```python
from build123d import *

# Parameters (mm, degrees)
BOSS_EXTRUDE1_DEPTH                             = 6.35
FILLET1_R                                       = 10
CSK_FOR_M4_FLAT_HEAD_MACHINE_SCREW1_D           = 4.5
CSK_FOR_M4_FLAT_HEAD_MACHINE_SCREW1_DEPTH       = 41.15
CSK_FOR_M4_FLAT_HEAD_MACHINE_SCREW1_CSINK_D     = 9.4
CSK_FOR_M4_FLAT_HEAD_MACHINE_SCREW1_CSINK_ANGLE = 90
CSK_FOR_M4_FLAT_HEAD_MACHINE_SCREW1_TIP         = 1.351936393
SKETCH5_R                                       = 23.5
CUT_EXTRUDE1_DEPTH                              = 91.971053662
FILLET2_R                                       = 5


with BuildPart() as part:
    # Sketch1 → Boss-Extrude1 (new body)
    with BuildSketch(Plane(origin=(0, 0, 0), x_dir=(1, 0, 0), z_dir=(0, 1, 0))):
        with BuildLine():
            ThreePointArc((-15.208520638, -24.071794541), (-40.946506862, -5.668779355), (-50.8, 24.398205459))
            Line((-50.8, 24.398205459), (-50.8, -73.601794541))
            Line((-50.8, -73.601794541), (-30.8, -73.601794541))
            Line((-30.8, -73.601794541), (-30.8, -24.071794541))
            Line((-30.8, -24.071794541), (-15.208520638, -24.071794541))
        make_face()
        with BuildLine():
            Line((0, 24.398205459), (-50.8, 24.398205459))
            ThreePointArc((-50.8, 24.398205459), (-40.946506862, -5.668779355), (-15.208520638, -24.071794541))
            Line((-15.208520638, -24.071794541), (0, -24.071794541))
            Line((0, -24.071794541), (0, 24.398205459))
        make_face()
        with BuildLine():
            Line((50.8, 24.398205459), (0, 24.398205459))
            Line((0, 24.398205459), (0, -24.071794541))
            Line((0, -24.071794541), (15.208520638, -24.071794541))
            ThreePointArc((15.208520638, -24.071794541), (40.946506862, -5.668779355), (50.8, 24.398205459))
        make_face()
        with BuildLine():
            ThreePointArc((50.8, 24.398205459), (0, 75.198205459), (-50.8, 24.398205459))
            Line((-50.8, 24.398205459), (0, 24.398205459))
            Line((0, 24.398205459), (50.8, 24.398205459))
        make_face()
        with BuildLine():
            Line((50.8, -73.601794541), (50.8, 24.398205459))
            ThreePointArc((50.8, 24.398205459), (40.946506862, -5.668779355), (15.208520638, -24.071794541))
            Line((15.208520638, -24.071794541), (30.8, -24.071794541))
            Line((30.8, -24.071794541), (30.8, -73.601794541))
            Line((30.8, -73.601794541), (50.8, -73.601794541))
        make_face()
    extrude(amount=BOSS_EXTRUDE1_DEPTH)

    # Fillet1
    fillet1_edges = [part.edges().sort_by_distance(p)[0] for p in [
        (-30.8, 3.175, 24.071794541),
        (30.8, 3.175, 24.071794541),
    ]]
    fillet(fillet1_edges, radius=FILLET1_R)

    # CSK for M4 Flat Head Machine Screw1
    with Locations(Plane.XZ):
        with Locations((44.261727213, -14.295755058), (-44.45, 65.601794541), (44.45, 65.601794541), (-44.45, 21.601794541), (44.45, 21.601794541), (19.698321756, 16.505781144), (-19.698321756, 16.505781144), (-44.261727213, -14.295755058), (-35.495149304, -52.704642464), (0, -69.798205459), (35.495149304, -52.704642464)):
            CounterSinkHole(CSK_FOR_M4_FLAT_HEAD_MACHINE_SCREW1_D / 2, CSK_FOR_M4_FLAT_HEAD_MACHINE_SCREW1_CSINK_D / 2, depth=CSK_FOR_M4_FLAT_HEAD_MACHINE_SCREW1_DEPTH, counter_sink_angle=CSK_FOR_M4_FLAT_HEAD_MACHINE_SCREW1_CSINK_ANGLE)
            with Locations((0, 0, -(CSK_FOR_M4_FLAT_HEAD_MACHINE_SCREW1_DEPTH + CSK_FOR_M4_FLAT_HEAD_MACHINE_SCREW1_TIP / 2))):  # 118° drill point
                Cone(0, CSK_FOR_M4_FLAT_HEAD_MACHINE_SCREW1_D / 2, CSK_FOR_M4_FLAT_HEAD_MACHINE_SCREW1_TIP, mode=Mode.SUBTRACT)

    # Sketch5 → Cut-Extrude1 (cut, through all)
    with BuildSketch(Plane.XZ):
        with Locations(Location((0, -24.398205459, 0), (0, 0, 270))):
            Circle(SKETCH5_R)
    extrude(amount=-CUT_EXTRUDE1_DEPTH, mode=Mode.SUBTRACT)

    # Fillet2
    fillet2_edges = [part.edges().sort_by_distance(p)[0] for p in [
        (-30.8, 3.175, 73.601794541),
        (-50.8, 3.175, 73.601794541),
        (50.8, 3.175, 73.601794541),
        (30.8, 3.175, 73.601794541),
    ]]
    fillet(fillet2_edges, radius=FILLET2_R)


solid = part.part
```
Part model, mm, in its own coordinate system. A direction names the side the tool comes from. Give positions to 0.01 mm unless a question says otherwise; leave off trailing zeros. Loops run counter-clockwise (first coordinate to the right, second up) from the corner with the lowest first, then second, coordinate; pieces in that order, holes last. Notation, with made-up numbers: M 43,-29.75 L 94,-29.75 A14 ccw 94,-4.75 Z; hole C 74,78 d7. An arc over 180 degrees is marked long. Return JSON: item names as keys, results as strings.
1) 3-axis set-ups, long thin cutter, end or side, ignore diameter. For faces 4 (the face through (27.79, 3.22, 26.92)), 5 (the face through (36.01, 2.33, -55.02)): which of +Z, -Z, +X, -X, +Y, -Y reach the whole face in a straight line?
Calculated:
{"face 4": "+Z, +Y, -Y", "face 5": "-Y"}
2) Saw through at C-C, the plane y = 4.75. Count the separate pieces of the cut face and the enclosed holes in it, then the cut area to 3 significant figures.
Calculated:
{"separate pieces": "1", "enclosed holes": "12", "area": "9,070 mm2"}
3) Drill centre lines: line 1 (Z direction, x = -44.45, y = 5); line 2 (X direction, y = 4.5, z = 44.5); line 3 (X direction, y = 1.25, z = -25). Where is each one in solid material? Low to high.
Calculated:
{"line 1": "z = -48.99 to -16.54, -12.05 to 19.35, 23.85 to 63.35, 67.85 to 73.6", "line 2": "x = -50.8 to -30.8, 30.8 to 50.8", "line 3": "x = -50.8 to -23.49, 23.49 to 50.8"}
4) Saw through at D-D, the plane x = -12. List the corners of the cut face in (y, z), then the cut area to 3 significant figures.
Calculated:
{"outline": "M 0,-73.76 L 6.35,-73.76 L 6.35,-44.6 L 0,-44.6 Z; M 0,-4.19 L 6.35,-4.19 L 6.35,24.07 L 0,24.07 Z", "area": "365 mm2"}
5) Pull direction Z, two halves, no side cores. Call faces 1 (the face through (-46.34, 4.43, -15.16)), 2 (the face through (-27.95, 3.22, 27.08)), 3 (the face through (30.8, 3, 51)): released by +Z, released by -Z, zero draft, split by the parting line, or undercut.
Calculated:
{"face 1": "undercut", "face 2": "released by +Z", "face 3": "zero draft"}
6) Flat gauge pins, fed straight in: pin 1 Ø5 at (x, z) = (40.5, -60.5) entering from +Y; pin 2 Ø3 at (x, y) = (-33.5, 1.5) entering from -Z; pin 3 Ø1 at (y, z) = (4.5, -49) entering from -X; pin 4 Ø6 at (x, z) = (35.5, -52.7) entering from -Y. Where does each tip first touch, or does it go through?
Calculated:
{"pin 1": "passes through", "pin 2": "stops at z = -63.85", "pin 3": "stops at x = -44.72", "pin 4": "stops at y = 1.69"}
7) Saw through at A-A, the plane x = 0. List the corners of the cut face in (y, z), then the cut area to 3 significant figures.
Calculated:
{"outline": "M 0,-75.2 L 6.35,-75.2 L 6.35,-72.05 L 2.45,-72.05 L 0,-74.5 Z; M 0,-65.1 L 2.45,-67.55 L 6.35,-67.55 L 6.35,-47.9 L 0,-47.9 Z; M 0,-0.9 L 6.35,-0.9 L 6.35,24.07 L 0,24.07 Z", "area": "297 mm2"}
8) Saw through at B-B, the plane z = -31. List the corners of the cut face in (x, y).
Calculated:
{"outline": "M -50.37,0 L -22.55,0 L -22.55,6.35 L -50.37,6.35 Z; M 22.55,0 L 50.37,0 L 50.37,6.35 L 22.55,6.35 Z"}
